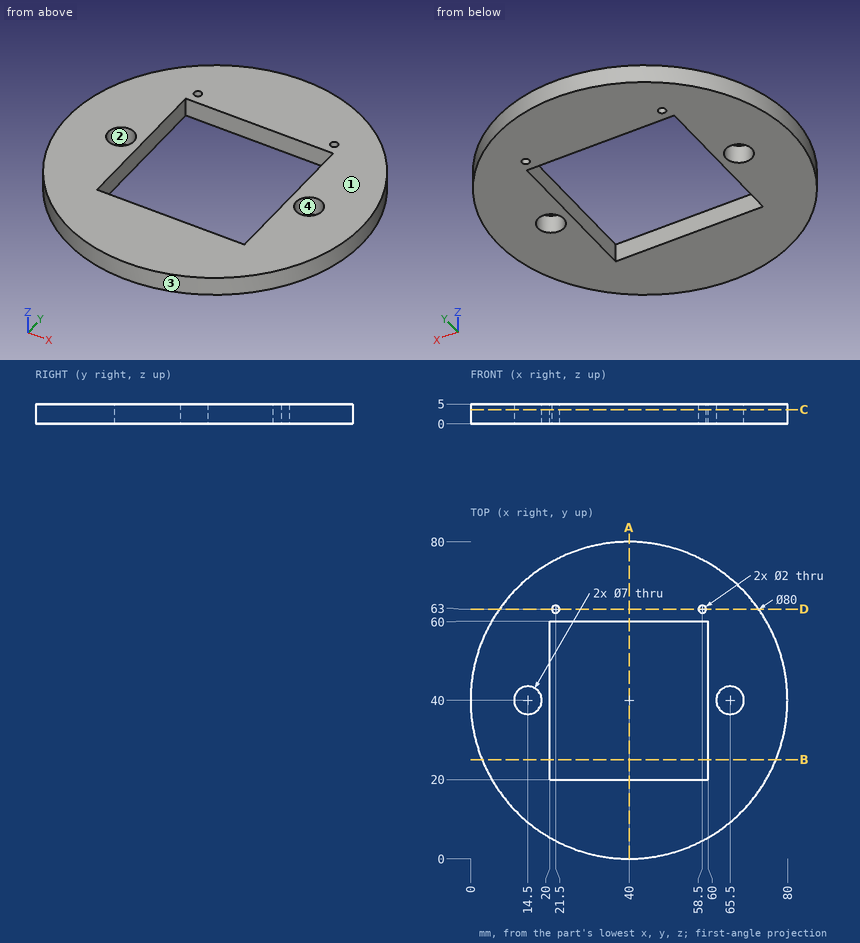
Answer from the drawing. Dimensions are ordinates in mm from the lowest x, y and z of the part. Give positions to 0.01 mm unless a question says otherwise; leave off trailing zeros. Loops run counter-clockwise (first coordinate to the right, second up) from the corner with the lowest first, then second, coordinate; pieces in that order, holes last.
Item 1: The part is cut by section A-A (x = 40). Write down the section's boundary in (y, z), and give its area (3 significant figures).
Item 2: Each of these flat-tipped pins is pushed along its axis until it touches: pin 1 Ø1.5 at (x, z) = (52, 1) entering from -Y; pin 2 Ø1.5 at (y, z) = (22, 1) entering from -X; pin 3 Ø2.5 at (y, z) = (43.5, 2.5) entering from -X; pin 4 Ø6.5 at (x, y) = (65.5, 40) entering from +Z. Where does it stop, or does it pass through?
Item 3: The part is cut by section D-D (y = 63). Write down the section's boundary in (x, z), and give its area (3 significant figures).
Item 4: The mould has two halves that part along Y. Classify the marked faces 1, 2, 3 and 4: released by +Y, released by -Y, zero draft, split by the parting line, or undercut.
Item 5: The part is cut by section B-B (y = 25). Write down the section's boundary in (x, z).
Item 6: The part is cut by section C-C (z = 3.55). Write down the section's boundary in (x, y), and give its area (3 significant figures).
Item 7: Find the intervals of material crossed by line 1 along Y through (x, z) = (58.5, 1.1); line 2 along X through (y, z) = (39.5, 3.1); line 3 along X through (y, z) = (30, 3.15), in increasing order.
Taken from the geometry:
1. outline: (0, 0) - (20, 0) - (20, 5) - (0, 5) - close; (60, 0) - (80, 0) - (80, 5) - (60, 5) - close
1. area: 200 mm2
2. pin 1: stops at y = 1.61
2. pin 2: stops at x = 3.91
2. pin 3: stops at x = 0.06
2. pin 4: passes through
3. outline: (7.27, 0) - (20.5, 0) - (20.5, 5) - (7.27, 5) - close; (22.5, 0) - (57.5, 0) - (57.5, 5) - (22.5, 5) - close; (59.5, 0) - (72.73, 0) - (72.73, 5) - (59.5, 5) - close
3. area: 307 mm2
4. face 1: zero draft
4. face 2: undercut
4. face 3: split by the parting line
4. face 4: undercut
5. outline: (2.92, 0) - (20, 0) - (20, 5) - (2.92, 5) - close; (60, 0) - (77.08, 0) - (77.08, 5) - (60, 5) - close
6. outline: circle Ø80 at (40, 40); hole circle Ø7 at (14.5, 40); hole (20, 20) - (60, 20) - (60, 60) - (20, 60) - close; hole circle Ø2 at (21.5, 63); hole circle Ø2 at (58.5, 63); hole circle Ø7 at (65.5, 40)
6. area: 3,340 mm2
7. line 1: y = 4.54 to 20, 60 to 62, 64 to 75.46
7. line 2: x = 0 to 11.04, 17.96 to 20, 60 to 62.04, 68.96 to 80
7. line 3: x = 1.27 to 20, 60 to 78.73
